from build123d import *

# Parameters (mm, degrees)
BOSS_EXTRUDE1_DEPTH = 60
SKETCH3_R           = 3.25
CUT_EXTRUDE1_DEPTH  = 8
SKETCH4_R           = 2
CUT_EXTRUDE2_DEPTH  = 8
CUT_EXTRUDE3_REACH  = 50
SKETCH5_R           = 1.32
SKETCH6_R           = 3.25
CUT_EXTRUDE4_DEPTH  = 6


with BuildPart() as part:
    # Sketch1 → Boss-Extrude1 (new body)
    with BuildSketch(Plane.XY):
        Polygon((-48, 0), (-48, 10), (-40, 10), (-40, 2), (-8, 2), (-8, 10), (0, 10), (0, 0), align=None)
    extrude(amount=BOSS_EXTRUDE1_DEPTH)

    # Sketch3 → Cut-Extrude1 (cut)
    with BuildSketch(Plane(origin=(0, 10, 0), x_dir=(1, 0, 0), z_dir=(0, 1, 0))):
        with Locations((-44, -5)):
            Circle(SKETCH3_R)
        with Locations((-4, -5)):
            Circle(SKETCH3_R)
        with Locations((-4, -55)):
            Circle(SKETCH3_R)
        with Locations((-44, -55)):
            Circle(SKETCH3_R)
    extrude(amount=-CUT_EXTRUDE1_DEPTH, mode=Mode.SUBTRACT)

    # Sketch4 → Cut-Extrude2 (cut)
    with BuildSketch(Plane.XZ):
        with Locations((-44, 55)):
            Circle(SKETCH4_R)
        with Locations((-4, 55)):
            Circle(SKETCH4_R)
        with Locations((-4, 5)):
            Circle(SKETCH4_R)
        with Locations((-44, 5)):
            Circle(SKETCH4_R)
    extrude(amount=-CUT_EXTRUDE2_DEPTH, mode=Mode.SUBTRACT)

    # Sketch5 → Cut-Extrude3 (cut, up to next)
    with BuildSketch(Plane.ZY.offset(48), mode=Mode.PRIVATE) as cut_extrude3_sk1:
        with Locations((12.75, 6)):
            Circle(SKETCH5_R)
    cut_extrude3_tool1 = extrude(cut_extrude3_sk1.sketch, amount=-CUT_EXTRUDE3_REACH, mode=Mode.PRIVATE) & part.part
    add(cut_extrude3_tool1.solids().sort_by_distance((-48, 6, 12.75))[0], mode=Mode.SUBTRACT)
    # Sketch5 → Cut-Extrude3 (cut, up to next)
    with BuildSketch(Plane.ZY.offset(48), mode=Mode.PRIVATE) as cut_extrude3_sk2:
        with Locations((30, 6)):
            Circle(SKETCH5_R)
    cut_extrude3_tool2 = extrude(cut_extrude3_sk2.sketch, amount=-CUT_EXTRUDE3_REACH, mode=Mode.PRIVATE) & part.part
    add(cut_extrude3_tool2.solids().sort_by_distance((-48, 6, 30))[0], mode=Mode.SUBTRACT)
    # Sketch5 → Cut-Extrude3 (cut, up to next)
    with BuildSketch(Plane.ZY.offset(48), mode=Mode.PRIVATE) as cut_extrude3_sk3:
        with Locations((47.25, 6)):
            Circle(SKETCH5_R)
    cut_extrude3_tool3 = extrude(cut_extrude3_sk3.sketch, amount=-CUT_EXTRUDE3_REACH, mode=Mode.PRIVATE) & part.part
    add(cut_extrude3_tool3.solids().sort_by_distance((-48, 6, 47.25))[0], mode=Mode.SUBTRACT)

    # Sketch6 → Cut-Extrude4 (cut)
    with BuildSketch(Plane.ZY.offset(48)):
        with Locations((12.75, 6)):
            Circle(SKETCH6_R)
        with Locations((30, 6)):
            Circle(SKETCH6_R)
        with Locations((47.25, 6)):
            Circle(SKETCH6_R)
    extrude(amount=-CUT_EXTRUDE4_DEPTH, mode=Mode.SUBTRACT)


solid = part.part
The listing builds one solid part. Answer for the finished solid, in the listing's coordinates (mm). A direction names the side the tool comes from. Coordinates: 2 decimals unless noted, no trailing zeros. Write each loop counter-clockwise with the first axis right and the second up, starting at its lowest first coordinate (ties: lowest second). Pieces come first, ordered by that corner, then holes. Notation, with made-up numbers: (-17.75, 11) - (-3.75, 11) arc R17 cw to (-3.75, 21) - close; hole circle Ø10 at (-24, 83). An arc over 180 degrees is marked (long way). Put each result on its own line as item: value.
1. Find the intervals of material crossed by line 1 along X through (y, z) = (5.5, 55); line 2 along Z through (x, y) = (-4, 6); line 3 along X through (y, z) = (3.75, 51.5), in increasing order. Write a range as from..to.
Answer sheet:
line 1: x = -48..-47.25, -40.75..-40, -8..-7.25, -0.75..0
line 2: z = 0..1.75, 8.25..51.75, 58.25..60
line 3: x = -48..-40, -8..0
2. The part is cut by section A-A on x = -44. Give the vertices of the cut face in (y, z), plus the area to 3 significant figures.
Answer sheet:
outline: (0, 0) - (10, 0) - (10, 1.75) - (2, 1.75) - (2, 3) - (0, 3) - close; (0, 7) - (2, 7) - (2, 8.25) - (10, 8.25) - (10, 51.75) - (2, 51.75) - (2, 53) - (0, 53) - close; (0, 57) - (2, 57) - (2, 58.25) - (10, 58.25) - (10, 60) - (0, 60) - close; hole circle Ø6.5 at (6, 12.75); hole circle Ø6.5 at (6, 30); hole circle Ø6.5 at (6, 47.25)
area: 380 mm^2
3. A tool of negligible diameter and unlimited length cuts with its end or side. For faces 1 (the face through (-4.423, 6.056, 51.778)), 2 (the face through (-41.014, 5.494, 13.969)), 3 (the face through (-8, 6, 30)), from which of +Z, -Z, +X, -X, +Y, -Y can it reach the whole face along a straight path? Write none if from no direction.
Answer sheet:
face 1: +Y
face 2: -X
face 3: +Z, -Z, +Y
4. The part is cut by section B-B on z = 30. Give the vertices of the cut face in (x, y).
Answer sheet:
outline: (-48, 0) - (0, 0) - (0, 10) - (-8, 10) - (-8, 2) - (-40, 2) - (-40, 4.68) - (-42, 4.68) - (-42, 2.75) - (-48, 2.75) - close; (-48, 9.25) - (-42, 9.25) - (-42, 7.32) - (-40, 7.32) - (-40, 10) - (-48, 10) - close
5. The part is cut by section C-C on x = -4. Give the vertices of the cut face in (y, z).
Answer sheet:
outline: (0, 0) - (10, 0) - (10, 1.75) - (2, 1.75) - (2, 3) - (0, 3) - close; (0, 7) - (2, 7) - (2, 8.25) - (10, 8.25) - (10, 51.75) - (2, 51.75) - (2, 53) - (0, 53) - close; (0, 57) - (2, 57) - (2, 58.25) - (10, 58.25) - (10, 60) - (0, 60) - close
6. Flat-ended cylindrical pins translate along their axes: pin 1 Ø2 at (x, z) = (-45, 4.5) entering from +Y; pin 2 Ø4.5 at (x, z) = (-4, 55) entering from -Y; pin 3 Ø2 at (y, z) = (6, 12.75) entering from -X; pin 4 Ø5 at (y, z) = (6, 12.75) entering from -X. Find the tip coordinate at first contact, or state that the pin passes through.
Answer sheet:
pin 1: stops at y = 2
pin 2: stops at y = 0
pin 3: stops at x = -8
pin 4: stops at x = -42
7. Determine the mould class of faces 4 (the face through (-24, 2, 30)), 5 (the face through (-45, 6.1, 9.5)), 6 (the face through (-45.04, 6.98, 50.35)), 7 (the face through (-40, 8, 30)) for opening direction Y: pulls with the +Y half, pulls with the -Y half, needs draft (parallel to the pull), parting line crosses it, or undercut.
Answer sheet:
face 4: pulls with the +Y half
face 5: undercut
face 6: undercut
face 7: needs draft
8. The part is cut by section D-D on z = 5. Give the vertices of the cut face in (x, y), plus the area to 3 significant figures.
Answer sheet:
outline: (-48, 0) - (-46, 0) - (-46, 2) - (-47.25, 2) - (-47.25, 10) - (-48, 10) - close; (-42, 0) - (-6, 0) - (-6, 2) - (-7.25, 2) - (-7.25, 10) - (-8, 10) - (-8, 2) - (-40, 2) - (-40, 10) - (-40.75, 10) - (-40.75, 2) - (-42, 2) - close; (-2, 0) - (0, 0) - (0, 10) - (-0.75, 10) - (-0.75, 2) - (-2, 2) - close
area: 104 mm^2
